Can you work these out from the model? Positions are in its coordinate system, mm. Round coordinates to 2 decimals unless told otherwise and drop trailing zeros. Loops run counter-clockwise (first coordinate to the right, second up) from the corner with the lowest first, then second, coordinate; pieces in that order, holes last.
from build123d import *

# Parameters (mm, degrees)
F1_DEPTH = 9.525


with BuildPart() as f1:
    # F0 (on Right) → F1 (new body)
    with BuildSketch(Plane.YZ):
        Polygon((-603.97613, 222.654683), (-603.97613, -82.145317), (-172.17613, -56.745317), (-172.17613, 248.054683), align=None)
    extrude(amount=F1_DEPTH)


with BuildPart() as f2_1:
    # F2: copy of F1
    add(f1.part.moved(Location((482.6, 0, 0))))


solid = f1.part
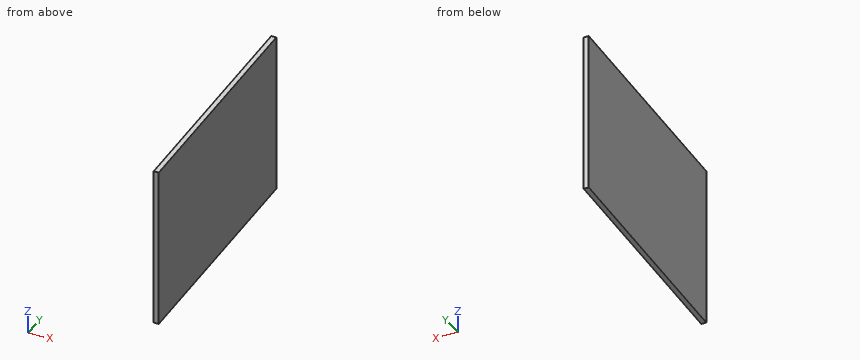
(1) If we section it at A-A, the plane x = 2.25: List the corners of the cut face in (y, z) for me.
Worked answers:
outline: (-603.98, -82.15) - (-172.18, -56.75) - (-172.18, 248.05) - (-603.98, 222.65) - close
(2) Will this pin go through, and if not, where does the flat tip stop? P1, Ø2, axis at x = 3, y = -471.5, coming from the -Z side.
Worked answers:
P1: stops at z = -74.41
(3) If I drill on line 1 (Z direction, x = 3.5, y = -411); line 2 (Z direction, x = 6.75, y = -550.5), over which ranges is the centre line in solid material (lowest first)?
Worked answers:
line 1: z = -70.79 to 234.01
line 2: z = -79 to 225.8
(4) If we section it at B-B, the plane y = -449: List the corners of the cut face in (x, z) for me (3 decimals), then the cut area to 3 significant figures.
Worked answers:
outline: (0, -73.029) - (9.525, -73.029) - (9.525, 231.771) - (0, 231.771) - close
area: 2,900 mm2
